```python
from build123d import *

# Parameters (mm, degrees)
EXTRUDE_1_DEPTH     = 3
EXTRUDE_2_DEPTH     = 10.3
EXTRUDE_3_DEPTH     = 1.8
FILLET_1_R          = 2
CUT_EXTRUDE_1_DEPTH = 2.5
CUT_EXTRUDE_2_REACH = 49.449
SKETCH_7_R          = 1.6
SKETCH_8_R          = 1.6
EXTRUDE_4_DEPTH     = 2.5
CHAMFER_1_SIZE      = 2.5
EXTRUDE_5_DEPTH     = 8


with BuildPart() as part:
    # Эскиз3 → Бобышка-Вытянуть1 (new body)
    with BuildSketch(Plane.XY):
        with BuildLine():
            Line((-35.402667816, -8), (-26.289419162, -8))
            ThreePointArc((-26.289419162, -8), (-23.789419162, -8.669872981), (-21.959292144, -10.5))
            Line((-21.959292144, -10.5), (-12, -27.75))
            Line((-12, -27.75), (-0.15, -27.75))
            Line((-0.15, -27.75), (-0.15, 27.75))
            Line((-0.15, 27.75), (-12, 27.75))
            Line((-12, 27.75), (-21.959292144, 10.5))
            ThreePointArc((-21.959292144, 10.5), (-23.789419162, 8.669872981), (-26.289419162, 8))
            Line((-26.289419162, 8), (-35.402667816, 8))
            Line((-35.402667816, 8), (-35.402667816, -8))
        make_face()
    extrude(amount=-EXTRUDE_1_DEPTH)

    # Эскиз4 → Бобышка-Вытянуть2 (add)
    with BuildSketch(Plane(origin=(0, 0, -3), x_dir=(-1, 0, 0), z_dir=(0, 0, -1))):
        with BuildLine():
            Line((12, -27.75), (0.15, -27.75))
            Line((0.15, -27.75), (0.15, -23.75))
            Line((0.15, -23.75), (9.690598923, -23.75))
            Line((9.690598923, -23.75), (12.609925056, -18.693578815))
            ThreePointArc((12.609925056, -18.693578815), (15.216591048, -16.5), (15.81295303, -13.145771625))
            Line((15.81295303, -13.145771625), (18.495190528, -8.5))
            ThreePointArc((18.495190528, -8.5), (21.789419162, -5.205771366), (26.289419162, -4))
            Line((26.289419162, -4), (35.402667816, -4))
            Line((35.402667816, -4), (35.402667816, -8))
            Line((35.402667816, -8), (26.289419162, -8))
            ThreePointArc((26.289419162, -8), (23.789419162, -8.669872981), (21.959292144, -10.5))
            Line((21.959292144, -10.5), (12, -27.75))
        make_face()
        with BuildLine():
            Line((26.289419162, 8), (35.402667816, 8))
            Line((35.402667816, 8), (35.402667816, 4))
            Line((35.402667816, 4), (26.289419162, 4))
            ThreePointArc((26.289419162, 4), (21.789419162, 5.205771366), (18.495190528, 8.5))
            Line((18.495190528, 8.5), (15.81295303, 13.145771625))
            ThreePointArc((15.81295303, 13.145771625), (15.216591048, 16.5), (12.609925056, 18.693578815))
            Line((12.609925056, 18.693578815), (9.690598923, 23.75))
            Line((9.690598923, 23.75), (0.15, 23.75))
            Line((0.15, 23.75), (0.15, 27.75))
            Line((0.15, 27.75), (12, 27.75))
            Line((12, 27.75), (21.959292144, 10.5))
            ThreePointArc((21.959292144, 10.5), (23.789419162, 8.669872981), (26.289419162, 8))
        make_face()
    extrude(amount=EXTRUDE_2_DEPTH)

    # Эскиз5 → Бобышка-Вытянуть3 (add)
    with BuildSketch(Plane(origin=(0, 0, -13.3), x_dir=(-1, 0, 0), z_dir=(0, 0, -1))):
        with BuildLine():
            Line((18.495190528, -8.5), (16.495190528, -11.964101615))
            Line((16.495190528, -11.964101615), (18.097337525, -12.889101615))
            Line((18.097337525, -12.889101615), (20.097337525, -9.425))
            ThreePointArc((20.097337525, -9.425), (22.714419162, -6.807918363), (26.289419162, -5.85))
            Line((26.289419162, -5.85), (32.402667816, -5.85))
            Line((32.402667816, -5.85), (32.402667816, -4))
            Line((32.402667816, -4), (26.289419162, -4))
            ThreePointArc((26.289419162, -4), (21.789419162, -5.205771366), (18.495190528, -8.5))
        make_face()
        with BuildLine():
            Line((32.402667816, 4), (26.289419162, 4))
            ThreePointArc((26.289419162, 4), (21.789419162, 5.205771366), (18.495190528, 8.5))
            Line((18.495190528, 8.5), (16.495190528, 11.964101615))
            Line((16.495190528, 11.964101615), (18.097337525, 12.889101615))
            Line((18.097337525, 12.889101615), (20.097337525, 9.425))
            ThreePointArc((20.097337525, 9.425), (22.714419162, 6.807918363), (26.289419162, 5.85))
            Line((26.289419162, 5.85), (32.402667816, 5.85))
            Line((32.402667816, 5.85), (32.402667816, 4))
        make_face()
    extrude(amount=EXTRUDE_3_DEPTH)

    # Скругление1
    fillet_1_edges = [part.edges().sort_by_distance(p)[0] for p in [
        (-30.846043489, 8, 0),
        (-23.789419162, 8.669872981, 0),
        (-16.979646072, 19.125, 0),
        (-16.979646072, -19.125, 0),
        (-23.789419162, -8.669872981, 0),
        (-30.846043489, -8, 0),
    ]]
    fillet(fillet_1_edges, radius=FILLET_1_R)

    # Эскиз6 → Вырез-Вытянуть1 (cut)
    with BuildSketch(Plane.XY):
        Polygon((-8.230652791, 24.4), (-9.904968571, 21.5), (-8.230652791, 18.6), (-4.882021229, 18.6), (-3.207705449, 21.5), (-4.882021229, 24.4), align=None)
        Polygon((-4.882021229, -24.4), (-8.230652791, -24.4), (-9.904968571, -21.5), (-8.230652791, -18.6), (-4.882021229, -18.6), (-3.207705449, -21.5), align=None)
    extrude(amount=-CUT_EXTRUDE_1_DEPTH, mode=Mode.SUBTRACT)

    # Эскиз7 → Вырез-Вытянуть2 (cut, up to next)
    with BuildSketch(Plane.XY, mode=Mode.PRIVATE) as cut_extrude_2_sk1:
        with Locations((-6.55633701, 21.5)):
            Circle(SKETCH_7_R)
    cut_extrude_2_tool1 = extrude(cut_extrude_2_sk1.sketch, amount=-CUT_EXTRUDE_2_REACH, mode=Mode.PRIVATE) & part.part
    # Эскиз7 → Вырез-Вытянуть2 (cut, up to next)
    with BuildSketch(Plane.XY, mode=Mode.PRIVATE) as cut_extrude_2_sk2:
        with Locations((-6.55633701, -21.5)):
            Circle(SKETCH_7_R)
    cut_extrude_2_tool2 = extrude(cut_extrude_2_sk2.sketch, amount=-CUT_EXTRUDE_2_REACH, mode=Mode.PRIVATE) & part.part
    add(cut_extrude_2_tool1.solids().sort_by_distance((-6.556337, 21.5, 0))[0], mode=Mode.SUBTRACT)
    add(cut_extrude_2_tool2.solids().sort_by_distance((-6.556337, -21.5, 0))[0], mode=Mode.SUBTRACT)

    # Эскиз8 → Бобышка-Вытянуть4 (add)
    # profile 1 of 2: a face of its own
    with BuildSketch(Plane(origin=(0, 0, -3), x_dir=(-1, 0, 0), z_dir=(0, 0, -1))):
        with BuildLine():
            Line((9.587425923, 19.75), (10.793712962, 21.839350439))
            Line((10.793712962, 21.839350439), (9.690598923, 23.75))
            Line((9.690598923, 23.75), (3.05633701, 23.75))
            Line((3.05633701, 23.75), (3.05633701, 21.5))
            ThreePointArc((3.05633701, 21.5), (5.650470352, 18.119259608), (9.587425923, 19.75))
        make_face()
        with Locations(Location((6.55633701, 21.5, 0), (0, 0, 180))):
            Circle(SKETCH_8_R, mode=Mode.SUBTRACT)
    # profile 2 of 2: a face of its own
    with BuildSketch(Plane(origin=(0, 0, -3), x_dir=(-1, 0, 0), z_dir=(0, 0, -1))):
        with BuildLine():
            Line((3.05633701, -23.75), (3.05633701, -21.5))
            ThreePointArc((3.05633701, -21.5), (5.650470352, -18.119259608), (9.587425923, -19.75))
            Line((9.587425923, -19.75), (10.793712962, -21.839350439))
            Line((10.793712962, -21.839350439), (9.690598923, -23.75))
            Line((9.690598923, -23.75), (3.05633701, -23.75))
        make_face()
        with Locations(Location((6.55633701, -21.5, 0), (0, 0, 180))):
            Circle(SKETCH_8_R, mode=Mode.SUBTRACT)
    extrude(amount=EXTRUDE_4_DEPTH)

    # Фаска1
    chamfer_1_edges = [part.edges().sort_by_distance(p)[0] for p in [
        (-10.190569442, -20.79467522, -3),
        (-3.05633701, -22.625, -3),
        (-5.650470352, -18.119259608, -3),
        (-3.05633701, 22.625, -3),
        (-10.190569442, 20.79467522, -3),
        (-5.650470352, 18.119259608, -3),
    ]]
    chamfer(chamfer_1_edges, length=CHAMFER_1_SIZE - 0.0001)  # a hair under: the kernel refuses the full size

    # Эскиз10 → Бобышка-Вытянуть5 (add)
    with BuildSketch(Plane.ZY.offset(35.402667816)):
        with BuildLine():
            Line((-10.3, 4), (-3, 4))
            Line((-3, 4), (-3, -4))
            Line((-3, -4), (-10.3, -4))
            Line((-10.3, -4), (-10.3, -3.9))
            ThreePointArc((-10.3, -3.9), (-6.4, 0), (-10.3, 3.9))
            Line((-10.3, 3.9), (-10.3, 4))
        make_face()
    extrude(amount=-EXTRUDE_5_DEPTH)


solid = part.part
```
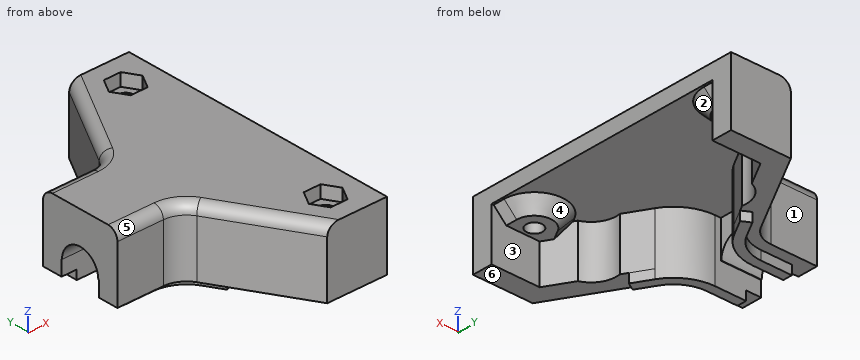
Here's how the part is built. I have some questions about the finished solid (model axes, mm). Face numbers are marked on the shaded views. A direction names the side the tool comes from. Coordinates: 2 decimals unless noted, no trailing zeros. Order: outer loops, then holes, each group sorted by start corner. A loop starts at its lowest first (then second) coordinate and runs counter-clockwise, first axis right, second up. Notation, with made-up numbers: (49.5, 42) -> (72.5, 42) arc R6 ccw to (72.5, 48) -> close; hole circle Ø3 at (-12, 44). An arc over 180 degrees is marked (long way). Return JSON: item names as keys, results as strings.
1) If we section it at C-C on z = -4: State how many separate pieces and enclosed holes the cut face has, plus the area to 3 significant figures.
Conclusion:
{"separate pieces": "1", "enclosed holes": "2", "area": "523 mm²"}
2) If I drill on probe 1 along Y at (x, z) = (-34, -12.25); probe 2 along X at (y, z) = (2, -3.25); probe 3 along Z at (x, y) = (-3, 6.5), over which ranges is the centre line in solid material (lowest first)?
Conclusion:
{"probe 1": "y = -8 to -4, 4 to 8", "probe 2": "x = -35.4 to -27.4", "probe 3": "z = -3 to 0"}
3) Thinking about a two-plate mould opening in Y: for the marked faces 4, 5 and 6, which applies, +Y half, -Y half, draft (parallel to the pull), parting line (faces both ways), or undercut?
Conclusion:
{"face 4": "undercut", "face 5": "-Y half", "face 6": "draft"}
4) On a 3-axis mill with a long thin cutter (end or side, diameter ignored), from which of +Z, -Z, +X, -X, +Y, -Y can I reach the whole of each face in a straight line? I mean the marked faces 1, 2 and 3. Say none if no direction works.
Conclusion:
{"face 1": "+Z, -Z, -X, +Y", "face 2": "-Z", "face 3": "-Z, +X"}
5) I'm going to push flat-ended pins straight in: P1, Ø1.7, axis at x = -6, y = 20.5, coming from the -Z side; P2, Ø1.5, axis at x = -32, y = 0, coming from the -Z side; P3, Ø1.7, axis at x = -7.5, y = 22, coming from the +Z side. Where does each tip first touch, or does it pass through?
Conclusion:
{"P1": "stops at z = -5.5", "P2": "stops at z = -6.47", "P3": "stops at z = -2.5"}
6) If we section it at B-B on y = 0: List the corners of the cut face in (x, z) for me, plus the area to 3 significant figures.
Conclusion:
{"outline": "(-35.4, -6.4) -> (-27.4, -6.4) -> (-27.4, -3) -> (-0.15, -3) -> (-0.15, 0) -> (-35.4, 0) -> close", "area": "133 mm²"}
7) If we section it at A-A on z = -12: List the corners of the cut face in (x, y) for me.
Conclusion:
{"outline": "(-35.4, -8) -> (-26.29, -8) arc R5 cw to (-21.96, -10.5) -> (-12, -27.75) -> (-0.15, -27.75) -> (-0.15, -23.75) -> (-9.69, -23.75) -> (-12.61, -18.69) arc R5 cw to (-15.81, -13.15) -> (-18.5, -8.5) arc R9 ccw to (-26.29, -4) -> (-35.4, -4) -> close; (-35.4, 4) -> (-26.29, 4) arc R9 ccw to (-18.5, 8.5) -> (-15.81, 13.15) arc R5 cw to (-12.61, 18.69) -> (-9.69, 23.75) -> (-0.15, 23.75) -> (-0.15, 27.75) -> (-12, 27.75) -> (-21.96, 10.5) arc R5 cw to (-26.29, 8) -> (-35.4, 8) -> close"}
